```python
from build123d import *

# Parameters (mm, degrees)
F0_W     = 25
F0_H     = 50
F1_DEPTH = 75
F3_DEPTH = 50
F5_DEPTH = 75


with BuildPart() as f1:
    # F0 (on Top) → F1 (new body)
    with BuildSketch(Plane.XY):
        with Locations((12.5, 25)):
            Rectangle(F0_W, F0_H)
    extrude(amount=F1_DEPTH)

    # F2 (on Top) → F3 (join)
    with BuildSketch(Plane.XY):
        Polygon((25, 50), (25, 0), (42.5, 0), (42.5, 15), (70, 15), (70, 10), (100, 10), (100, 40), (100, 50), (90, 50), align=None)
    extrude(amount=F3_DEPTH)

    # F4 (on face) → F5 (join)
    with BuildSketch(Plane(origin=(0, 0, 0), x_dir=(1, 0, 0), z_dir=(0, 0, -1))):
        Polygon((110, -10), (100, -10), (100, -50), (130, -50), (130, 20), (110, 20), align=None)
    extrude(amount=-F5_DEPTH)


solid = f1.part
```
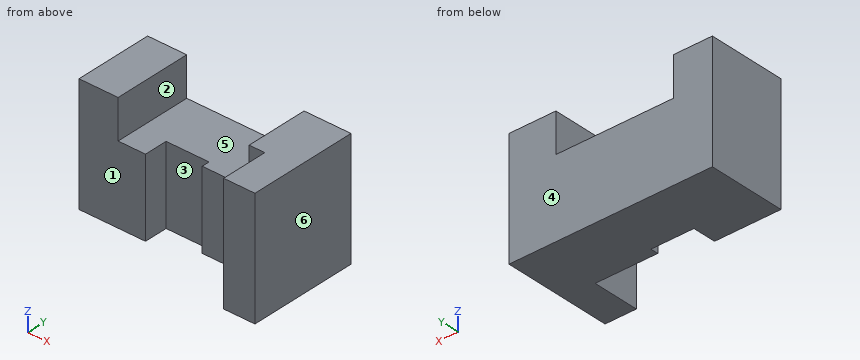
CAD build for the part. Positions are in the model's coordinates, mm. Face numbers are marked on the shaded views. A direction names the side the tool comes from. Round coordinates to 2 decimals unless told otherwise and drop trailing zeros. Loops run counter-clockwise (first coordinate to the right, second up) from the corner with the lowest first, then second, coordinate; pieces in that order, holes last. Notation, with made-up numbers: M 72,0 L 130,0 A24 cw 130,15 Z; hole C 69.5,34 d6. An arc over 180 degrees is marked long. Use a Markdown table: item, result. Add a question column.
(1) Drill centre lines: line 1 (X direction, y = 30, z = 66.5); line 2 (X direction, y = 12.5, z = 38); line 3 (Z direction, x = 52.5, y = 44.5). Where is each one in solid material? Low to high.
(2) Flat gauge pins, fed straight in: pin 1 (10 mm diameter, centred on x = 50, y = -5.5, fed in from -Z); pin 2 (1 mm diameter, centred on x = 92, y = 37.5, fed in from +Z); pin 3 (13 mm diameter, centred on x = 27.5, z = 34.5, fed in from -Y); pin 4 (10 mm diameter, centred on y = 33, z = 44.5, fed in from -X). Where does each tip first touch, or does it go through?
(3) Cut at C-C (z = 27). Give the cut face in (x, y).
(4) Which spindle directions (+Z, -Z, +X, -X, +Y, -Y) get a long thin tool onto all of the face, cutting with end or side? Do the marked faces 1, 2 and 3. Say none if no direction does.
(5) Pull direction X, two halves, no side cores. Call the marked faces 4, 5 and 6: +X half, -X half, draft (parallel to the pull), parting line (faces both ways), or undercut.
(6) Cut at D-D (y = 22). Give the cut face in (x, z).
(7) Cut at B-B (y = 2.5). Give the cut face in (x, z).
(8) Cut at A-A (z = 62). Give the cut face in (x, y), and give its area (3 significant figures).
Geometry says:
| question | item | result |
|---|---|---|
| 1 | line 1 | x = 0 to 25, 100 to 130 |
| 1 | line 2 | x = 0 to 42.5, 70 to 130 |
| 1 | line 3 | z = 0 to 50 |
| 2 | pin 1 | passes through |
| 2 | pin 2 | stops at z = 50 |
| 2 | pin 3 | stops at y = 0 |
| 2 | pin 4 | stops at x = 0 |
| 3 | outline | M 0,0 L 42.5,0 L 42.5,15 L 70,15 L 70,10 L 110,10 L 110,-20 L 130,-20 L 130,50 L 0,50 Z |
| 4 | face 1 | +Z, -Z, -X, -Y |
| 4 | face 2 | +Z, +Y, -Y |
| 4 | face 3 | +Z, -Z, -Y |
| 5 | face 4 | draft |
| 5 | face 5 | undercut |
| 5 | face 6 | +X half |
| 6 | outline | M 0,0 L 130,0 L 130,75 L 100,75 L 100,50 L 25,50 L 25,75 L 0,75 Z |
| 7 | outline | M 0,0 L 42.5,0 L 42.5,50 L 25,50 L 25,75 L 0,75 Z; M 110,0 L 130,0 L 130,75 L 110,75 Z |
| 8 | outline | M 0,0 L 25,0 L 25,50 L 0,50 Z; M 100,10 L 110,10 L 110,-20 L 130,-20 L 130,50 L 100,50 Z |
| 8 | area | 3,050 mm² |
